from build123d import *

# Parameters (mm, degrees)
F1_DEPTH = 66.5
F3_DEPTH = 2
F5_DEPTH = 2


with BuildPart() as f1:
    # F0 (on Front) → F1 (new body)
    with BuildSketch(Plane.XZ):
        Polygon((9.1355, 50), (0, 50), (-9.1355, 50), (-9.1355, 47), (-40, 16), (-40, 0), (0, 0), (40, 0), (40, 16), (9.1355, 47), align=None)
        Polygon((-6.7035206594, 44.8390617967), (0, 45.9953211248), (4.56775, 45.9953211248), (36.9867831469, 14.5120471716), (36.9867831469, 3.7666528951), (-36.0103435814, 3.7666528951), (-36.0103435814, 15.0574101135), align=None, mode=Mode.SUBTRACT)
    extrude(amount=F1_DEPTH)

    # F2 (on face) → F3 (join)
    with BuildSketch(Plane.XZ.offset(66.5)):
        Polygon((9.1355, 50), (-9.1355, 50), (-9.1355, 47), (-40, 16), (-40, 0), (40, 0), (40, 16), (9.1355, 47), align=None)
    extrude(amount=F3_DEPTH)

    # F4 (on face) → F5 (join)
    with BuildSketch(Plane(origin=(0, 0, 0), x_dir=(-1, 0, 0), z_dir=(0, 1, 0))):
        Polygon((9.1355, 50), (-9.1355, 50), (-9.1355, 47), (-40, 16), (-40, 0), (40, 0), (40, 16), (9.1355, 47), align=None)
    extrude(amount=-F5_DEPTH)


solid = f1.part
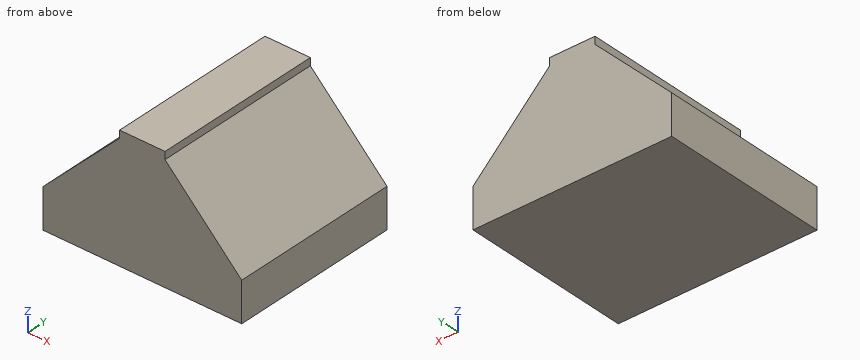
Source: CAD feature listing. Evaluate the final solid. Frame: model axes, mm. Coordinates: 2 decimals unless noted, no trailing zeros. Loops run counter-clockwise (first coordinate to the right, second up) from the corner with the lowest first, then second, coordinate; pieces in that order, holes last. Notation, with made-up numbers: (56.25, -10.5) - (115.25, -10.5) arc R22 ccw to (115.25, 5.5) - close; hole circle Ø8 at (67, 82.25). An arc over 180 degrees is marked (long way). One line per item, written item: value. Start each with the question number.
1. Ray query, L1, parallel to X at y = -52, z = 11.5; L2, parallel to Y at x = 14, z = 31.5; L3, parallel to Z at x = 2, y = -54. Return the intervals inside material, ascending.
2. Section B-B (y = -56). Return the cut outline in (x, z), and give its area (3 significant figures).
3. Section C-C (x = 11.5). Return the cut outline in (y, z), and give its area (3 significant figures).
4. Section A-A (z = 13.5). Return the cut outline in (x, y), and give its area (3 significant figures).
5. Contact query for flat-ended pins moving along their axis: P1, Ø4, axis at y = -45.5, z = 21, coming from the +X side; P2, Ø5, axis at x = 14, y = -39, coming from the +Z side; P3, Ø0.9, axis at y = -40.5, z = 49, coming from the -X side. Output: stop coordinate, or through.
Verdict:
1. L1: x = -40 to -36.01, 36.99 to 40
1. L2: y = -68.5 to -66.5, -2 to 0
1. L3: z = 0 to 3.77, 46 to 50
2. outline: (-40, 0) - (40, 0) - (40, 16) - (9.14, 47) - (9.14, 50) - (-9.14, 50) - (-9.14, 47) - (-40, 16) - close; hole (-36.01, 3.77) - (36.99, 3.77) - (36.99, 14.51) - (4.57, 46) - (0, 46) - (-6.7, 44.84) - (-36.01, 15.06) - close
2. area: 760 mm2
3. outline: (-68.5, 0) - (0, 0) - (0, 44.63) - (-68.5, 44.63) - close; hole (-66.5, 3.77) - (-2, 3.77) - (-2, 39.26) - (-66.5, 39.26) - close
3. area: 767 mm2
4. outline: (-40, -68.5) - (40, -68.5) - (40, 0) - (-40, 0) - close; hole (-36.01, -66.5) - (36.99, -66.5) - (36.99, -2) - (-36.01, -2) - close
4. area: 772 mm2
5. P1: stops at x = 37.01
5. P2: stops at z = 44.63
5. P3: stops at x = -9.14
